The listing builds one solid part. Answer for the finished solid, in the listing's coordinates (mm). Give positions to 0.01 mm unless a question says otherwise; leave off trailing zeros. Order: outer loops, then holes, each group sorted by start corner. A loop starts at its lowest first (then second) coordinate and runs counter-clockwise, first axis right, second up.
```python
from build123d import *

# Parameters (mm, degrees)
ESQUISSE1_W             = 42
ESQUISSE1_H             = 20
BASE_EXTRUSION_DEPTH    = 125
ENL_V_MAT_EXTRU_1_REACH = 135.375
ESQUISSE2_R             = 3.25
ESQUISSE3_R             = 3.375
ENL_V_MAT_EXTRU_2_DEPTH = 25


with BuildPart() as part:
    # Esquisse1 → Base-Extrusion (new body)
    with BuildSketch(Plane.XY):
        with Locations((21, 10)):
            Rectangle(ESQUISSE1_W, ESQUISSE1_H)
    extrude(amount=BASE_EXTRUSION_DEPTH)

    # Esquisse2 → Enlèv. mat.-Extru.1 (cut, up to next)
    with BuildSketch(Plane(origin=(0, 20, 0), x_dir=(-1, 0, 0), z_dir=(0, 1, 0)), mode=Mode.PRIVATE) as enl_v_mat_extru_1_sk1:
        with Locations(Location((-10, 10, 0), (0, 0, 90))):
            Circle(ESQUISSE2_R)
    enl_v_mat_extru_1_tool1 = extrude(enl_v_mat_extru_1_sk1.sketch, amount=-ENL_V_MAT_EXTRU_1_REACH, mode=Mode.PRIVATE) & part.part
    # Esquisse2 → Enlèv. mat.-Extru.1 (cut, up to next)
    with BuildSketch(Plane(origin=(0, 20, 0), x_dir=(-1, 0, 0), z_dir=(0, 1, 0)), mode=Mode.PRIVATE) as enl_v_mat_extru_1_sk2:
        with Locations(Location((-32, 10, 0), (0, 0, 90))):
            Circle(ESQUISSE2_R)
    enl_v_mat_extru_1_tool2 = extrude(enl_v_mat_extru_1_sk2.sketch, amount=-ENL_V_MAT_EXTRU_1_REACH, mode=Mode.PRIVATE) & part.part
    # Esquisse2 → Enlèv. mat.-Extru.1 (cut, up to next)
    with BuildSketch(Plane(origin=(0, 20, 0), x_dir=(-1, 0, 0), z_dir=(0, 1, 0)), mode=Mode.PRIVATE) as enl_v_mat_extru_1_sk3:
        with Locations(Location((-10, 32, 0), (0, 0, 90))):
            Circle(ESQUISSE2_R)
    enl_v_mat_extru_1_tool3 = extrude(enl_v_mat_extru_1_sk3.sketch, amount=-ENL_V_MAT_EXTRU_1_REACH, mode=Mode.PRIVATE) & part.part
    # Esquisse2 → Enlèv. mat.-Extru.1 (cut, up to next)
    with BuildSketch(Plane(origin=(0, 20, 0), x_dir=(-1, 0, 0), z_dir=(0, 1, 0)), mode=Mode.PRIVATE) as enl_v_mat_extru_1_sk4:
        with Locations(Location((-32, 32, 0), (0, 0, 90))):
            Circle(ESQUISSE2_R)
    enl_v_mat_extru_1_tool4 = extrude(enl_v_mat_extru_1_sk4.sketch, amount=-ENL_V_MAT_EXTRU_1_REACH, mode=Mode.PRIVATE) & part.part
    add(enl_v_mat_extru_1_tool1.solids().sort_by_distance((10, 20, 10))[0], mode=Mode.SUBTRACT)
    add(enl_v_mat_extru_1_tool2.solids().sort_by_distance((32, 20, 10))[0], mode=Mode.SUBTRACT)
    add(enl_v_mat_extru_1_tool3.solids().sort_by_distance((10, 20, 32))[0], mode=Mode.SUBTRACT)
    add(enl_v_mat_extru_1_tool4.solids().sort_by_distance((32, 20, 32))[0], mode=Mode.SUBTRACT)

    # Esquisse3 → Enlèv. mat.-Extru.2 (cut)
    with BuildSketch(Plane.XY.offset(125)):
        with Locations((10, 10)):
            Circle(ESQUISSE3_R)
        with Locations((32, 10)):
            Circle(ESQUISSE3_R)
    extrude(amount=-ENL_V_MAT_EXTRU_2_DEPTH, mode=Mode.SUBTRACT)


solid = part.part
```
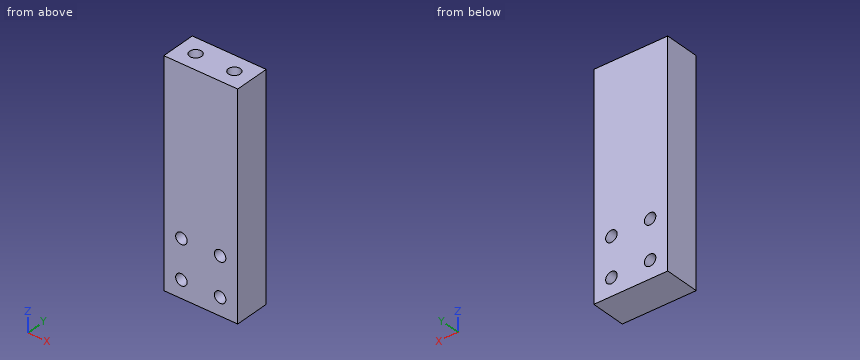
1) Straight lines are drawn through the part: probe 1 along X at (y, z) = (14.5, 32); probe 2 along Y at (x, z) = (32, 114) (3 decimals); probe 3 along Z at (x, y) = (30, 9.25). For each, find the intervals that lie inside material, in ascending order.
Geometry says:
probe 1: x = 0 to 6.75, 13.25 to 28.75, 35.25 to 42
probe 2: y = 0 to 6.625, 13.375 to 20
probe 3: z = 0 to 7.44, 12.56 to 29.44, 34.56 to 100
2) Find section B-B (x = 10). Write down the section's boundary in (y, z) (3 decimals), then the cut area to 3 significant figures.
Geometry says:
outline: (0, 0) - (20, 0) - (20, 6.75) - (0, 6.75) - close; (0, 13.25) - (20, 13.25) - (20, 28.75) - (0, 28.75) - close; (0, 35.25) - (20, 35.25) - (20, 125) - (13.375, 125) - (13.375, 100) - (6.625, 100) - (6.625, 125) - (0, 125) - close
area: 2,070 mm2
3) Find section D-D (y = 10). Write down the section's boundary in (x, z) (3 decimals).
Geometry says:
outline: (0, 0) - (42, 0) - (42, 125) - (35.375, 125) - (35.375, 100) - (28.625, 100) - (28.625, 125) - (13.375, 125) - (13.375, 100) - (6.625, 100) - (6.625, 125) - (0, 125) - close; hole circle Ø6.5 at (10, 10); hole circle Ø6.5 at (10, 32); hole circle Ø6.5 at (32, 10); hole circle Ø6.5 at (32, 32)
4) Given P1, Ø8, axis at y = 6.5, z = 88.5, coming from the -X side; P2, Ø2, axis at x = 9.5, y = 8.5, coming from the +Z side, each flat-ended and moving along its own axis, determine where each tip first touches the part or whether it passes through.
Geometry says:
P1: stops at x = 0
P2: stops at z = 100
5) Find section C-C (y = 4.5). Write down the section's boundary in (x, z), then the cut area to 3 significant figures.
Geometry says:
outline: (0, 0) - (42, 0) - (42, 125) - (0, 125) - close; hole circle Ø6.5 at (10, 10); hole circle Ø6.5 at (10, 32); hole circle Ø6.5 at (32, 10); hole circle Ø6.5 at (32, 32)
area: 5,120 mm2
6) Find section A-A (z = 10). Write down the section's boundary in (x, y).
Geometry says:
outline: (0, 0) - (6.75, 0) - (6.75, 20) - (0, 20) - close; (13.25, 0) - (28.75, 0) - (28.75, 20) - (13.25, 20) - close; (35.25, 0) - (42, 0) - (42, 20) - (35.25, 20) - close
